Autodesk Inventor part; units mm, degrees
ref_plane "YZ Plane" through (0, 0, 0) normal (1, 0, 0) x (0, 1, 0)
ref_plane "XZ Plane" through (0, 0, 0) normal (0, 1, 0) x (-1, 0, 0)
ref_plane "XY Plane" through (0, 0, 0) normal (0, 0, 1) x (1, 0, 0)
sketch "Sketch1" plane through (0, 0, 0) normal (0, 0, 1) x (1, 0, 0)
  line L0 (0, 0) -> (25, 0)
  line L1 (25, 0) -> (25, 40)
  line L2 (25, 40) -> (0, 40)
  line L3 (0, 40) -> (0, 0)
  dimension "d1" = 25
  dimension "d2" = 40
  dimension "d3" = 25
extrude "Extrusion1" add sketch "Sketch1" against normal blind 30
sketch "Sketch2" plane through (25, 0, 0) normal (1, 0, 0) x (0, 0, -1)
  line L0 (0, 0) -> (30, 0)
  circle A0 centre (15, 6.56) radius 2.46
extrude "Extrusion2" cut sketch "Sketch2" against normal blind 30
sketch "Sketch3" plane through (0, 0, 0) normal (-1, 0, 0) x (0, 0, 1)
  line L0 (0, 0) -> (-30, 0)
  line L1 (-25.05, 0) -> (-4.95, 0)
  line L2 (-4.95, 0) -> (-4.95, 33.12)
  line L3 (-4.95, 33.12) -> (-25.05, 33.12)
  line L4 (-25.05, 33.12) -> (-25.05, 0)
  dimension "d11" = 20.1
extrude "Extrusion3" cut sketch "Sketch3" against normal blind 20
sketch "Sketch4" plane through (0, 0, 0) normal (0, -1, 0) x (1, 0, 0)
  line L0 (20, -4.95) -> (20, -25.05)
  line L1 (20, -15) -> (25, -15)
  line L2 (25, 0) -> (25, -30)
  line L3 (20, -8.025) -> (25, -8.025)
  line L4 (25, -8.025) -> (25, -21.975)
  line L5 (25, -21.975) -> (20, -21.975)
  line L6 (20, -21.975) -> (20, -8.025)
  line L7 (20, -8.025) -> (25, -21.975) construction
  line L8 (25, -8.025) -> (20, -21.975) construction
  line L9 (25, -12.54) -> (25, -17.46)
  point P0 (0, 0)
  point P1 (22.5, -15)
  dimension "d14" = 13.95
extrude "Extrusion4" add sketch "Sketch4" along normal blind 15
sketch "Sketch5" plane through (20, 0, 0) normal (-1, 0, 0) x (0, 0, 1)
  circle A0 centre (-15, 6.56) radius 2.46
  circle A1 centre (-15, 6.56) radius 4.7025
  circle A2 centre (-15, 6.56) radius 2.46
  circle A3 centre (-15, 6.56) radius 2.46
  point P0 (0, 0)
  dimension "d17" = 9.405
extrude "Extrusion5" cut sketch "Sketch5" against normal blind 2.1
sketch "Sketch6" plane through (25, 0, 0) normal (1, 0, 0) x (0, 0, -1)
  circle A0 centre (15, 6.56) radius 4.7025
  line L0 (15, 6.56) -> (15, 23.56)
  circle A1 centre (15, 23.56) radius 2.46
  point P0 (0, 0)
  dimension "d20" = 17
  dimension "d21" = 4.92
extrude "Extrusion6" cut sketch "Sketch6" against normal blind 10 contours A1
sketch "Sketch7" plane through (20, 0, 0) normal (-1, 0, 0) x (0, 0, 1)
  circle A0 centre (-15, 23.56) radius 2.46
  circle A1 centre (-15, 23.56) radius 4.7025
  point P0 (0, 0)
  dimension "d24" = 9.405
extrude "Extrusion7" cut sketch "Sketch7" against normal blind 2.1
sketch "Sketch9" plane through (25, 0, 0) normal (1, 0, 0) x (0, 0, -1)
  circle A0 centre (15, 6.56) radius 2.46
  circle A1 centre (15, 6.56) radius 2.46
  circle A2 centre (15, 23.56) radius 2.46
  circle A3 centre (15, 23.56) radius 2.46
  line L0 (30, 40) -> (30, 0)
  line L1 (30, 0) -> (30, 40)
  line L2 (30, 40) -> (0, 40)
  line L3 (0, 40) -> (0, 0)
  line L4 (0, 0) -> (8.025, 0)
  line L5 (21.975, 0) -> (21.975, -15)
  line L6 (21.975, -15) -> (8.025, -15)
  line L7 (8.025, -15) -> (8.025, 0)
  line L8 (0, 0) -> (8.025, 0)
  line L9 (21.975, 0) -> (30, 0)
extrude "Extrusion8" add sketch "Sketch9" along normal blind 5
sketch "Sketch10" plane through (0, 40, 0) normal (0, 1, 0) x (1, 0, 0)
  line L0 (0, 30) -> (30, 30)
  line L1 (30, 0) -> (0, 0)
  line L2 (0, 30) -> (30, 30)
  line L3 (30, 30) -> (30, 0)
  line L4 (30, 0) -> (0, 0)
  line L5 (0, 0) -> (0, 30)
extrude "Extrusion9" add sketch "Sketch10" along normal blind 30
sketch "Sketch12" plane through (30, 0, 0) normal (1, 0, 0) x (0, 0, -1)
  circle A0 centre (15, 6.56) radius 2.46
  line L0 (15, 6.56) -> (15, 15.06)
  circle A1 centre (15, 15.06) radius 2.525
  point P0 (0, 0)
  dimension "d31" = 8.5
  dimension "d33" = 5.05
extrude "Extrusion10" cut sketch "Sketch12" against normal blind 30 contours A1
sketch "Sketch14" plane through (0, 0, 0) normal (0, 0, 1) x (1, 0, 0)
  line L0 (30, 70) -> (0, 70)
  line L1 (0, 70) -> (0, 85)
  line L2 (30, 0) -> (30, 70)
  line L3 (30, 118) -> (30, 70)
  line L4 (30, 105) -> (30, 100)
  line L5 (-12, 133) -> (15, 133)
  line L6 (-7, 130.5) -> (-12, 133)
  line L7 (-7, 130.5) -> (-2, 116.5)
  line L8 (-7, 102.5) -> (-12, 100)
  line L9 (-7, 102.5) -> (-2, 116.5)
  line L10 (30, 118) -> (15, 133)
  line L11 (0, 100) -> (-12, 100)
  line L12 (0, 100) -> (0, 85)
  point P0 (0, 0)
  dimension "d79" = 12
extrude "Extrusion12" add sketch "Sketch14" against normal blind 30
sketch "Sketch15" plane through (0, 0, -25.05) normal (-1, 0, 0) x (0, 0, 1)
  line L0 (0, 33.12) -> (20.1, 33.12)
  line L1 (20.1, 33.12) -> (20.1, 0)
  line L2 (0, 33.12) -> (20.1, 33.12)
  line L3 (20.1, 33.12) -> (20.1, 31.1)
  line L4 (20.1, 31.1) -> (0, 31.1)
  line L5 (0, 31.1) -> (0, 33.12)
  point P0 (25.05, 0)
  dimension "d57" = 2.02
extrude "Extrusion13" add sketch "Sketch15" against normal blind 20
properties part number "28mm_x_30mm"
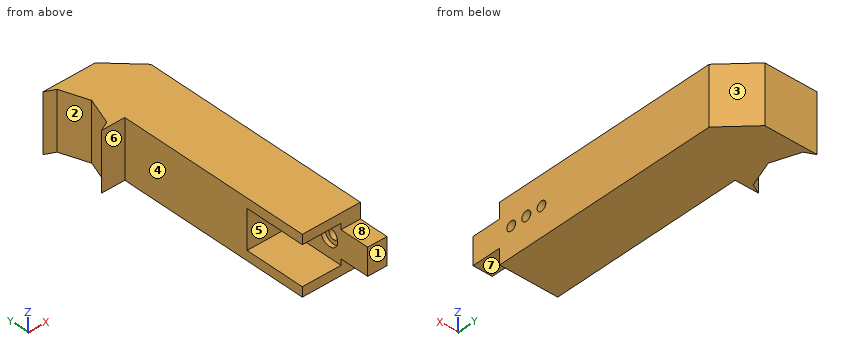
Input: part model. Units: mm. Frame: model coordinates. Face numbers are marked on the shaded views. A direction names the side the tool comes from. Coordinates: 2 decimals unless noted, no trailing zeros. Order: outer loops, then holes, each group sorted by start corner. A loop starts at its lowest first (then second) coordinate and runs counter-clockwise, first axis right, second up. Notation, with made-up numbers: M 28,-26.75 L 57,-26.75 A31 cw 57,5.25 Z; hole C 4.5,-13 d10. An arc over 180 degrees is marked long. Write item = value, one per line. Start each with the question number.
(1) First-contact query: P1, Ø4, axis at x = 8, z = -25.5, coming from the -Y side; P2, Ø4, axis at y = 36.5, z = -6, coming from the -X side; P3, Ø3, axis at x = 23.5, y = -9, coming from the -Z side (3 decimals). Flat tips, straight axial feed; report the tip coordinate or a pass-through.
(2) Section D-D on z = -27. Output: boundary loops of the cut face in (x, y).
(3) Section A-A on z = -15. Give the number of separate pieces and of enclosed holes in the cut face, and give its area (3 significant figures).
(4) Line query: line 1 along Z through (x, y) = (24.5, 23.56); line 2 along Z through (x, y) = (4.5, 7.5); line 3 along Y through (x, z) = (27.25, -15) (3 decimals). Output: solid intervals per line, ascending. Write a range as [from, to].
(5) Section B-B on y = 6.56. Output: boundary loops of the cut face in (x, z), and give its area (3 significant figures).
(6) Pull-direction query (Y, two-part tool) for the marked faces 1, 2, 3 and 4; classes: released by +Y, released by -Y, zero draft, split by the parting line, or undercut.
(7) Reachability of the marked faces 5, 6, 7 and 8 from +Z, -Z, +X, -X, +Y, -Y: full face, straight path, thin tool, end or side. Return the list, or none.
(8) Section C-C on x = 13. Output: boundary loops of the cut face in (y, z), and give its area (3 significant figures).
Result set:
q1.P1 = 0
q1.P2 = 0
q1.P3 = -21.975
q2.outline = M -12,100 L 0,100 L 0,0 L 30,0 L 30,118 L 15,133 L -12,133 L -7,130.5 L -2,116.5 L -7,102.5 Z
q3.separate_pieces = 4
q3.enclosed_holes = 0
q3.area = 3,410 mm²
q4.line_1 = [-30, -17.46], [-12.54, 0]
q4.line_2 = [-30, -25.05], [-4.95, 0]
q4.line_3 = [-15, 4.1], [9.02, 12.535], [17.585, 21.1], [26.02, 120.75]
q5.outline = M 0,-30 L 30,-30 L 30,-17.46 L 22.1,-17.46 L 22.1,-19.7 L 20,-19.7 L 20,-25.05 L 0,-25.05 Z; M 0,-4.95 L 20,-4.95 L 20,-10.3 L 22.1,-10.3 L 22.1,-12.54 L 30,-12.54 L 30,0 L 0,0 Z
q5.area = 439 mm²
q6.face_1 = released by -Y
q6.face_2 = undercut
q6.face_3 = released by +Y
q6.face_4 = zero draft
q7.face_5 = -X, -Y
q7.face_6 = +Z, -Z, -X, -Y
q7.face_7 = -Z, +X, -X, -Y
q7.face_8 = +Z, +X, -X, -Y
q8.outline = M 0,-30 L 133,-30 L 133,0 L 0,0 L 0,-4.95 L 31.1,-4.95 L 31.1,-25.05 L 0,-25.05 Z
q8.area = 3,360 mm²
